```python
from build123d import *

# Parameters (mm, degrees)
PAD_DEPTH    = 5
SKETCH002_W  = 180
SKETCH002_H  = 5
PAD002_DEPTH = 5
PAD003_DEPTH = 10


with BuildPart() as part:
    # Sketch → Pad (new body)
    with BuildSketch(Plane.XY):
        with BuildLine():
            Line((0, 0), (-11.5, 0))
            ThreePointArc((-13.5, 2), (-12.914214, 0.585786), (-11.5, 0))
            Line((-13.5, 2), (-13.5, 7))
            ThreePointArc((-12, 7), (-12.75, 7.75), (-13.5, 7))
            Line((-12, 7), (-12, 3))
            ThreePointArc((-12, 3), (-11.707107, 2.292893), (-11, 2))
            Line((-11, 2), (-3, 2))
            ThreePointArc((-3, 2), (-2.292893, 2.292893), (-2, 3))
            Line((-2, 8), (-2, 3))
            ThreePointArc((-2, 8), (-2.292893, 8.707107), (-3, 9))
            Line((-3, 9), (-9, 9))
            ThreePointArc((-9, 11), (-10, 10), (-9, 9))
            Line((0, 11), (-9, 11))
            Line((0, 11), (0, 0))
        make_face()
    extrude(amount=PAD_DEPTH)

    # Sketch002 → Pad002 (join)
    with BuildSketch(Plane.XY):
        with Locations((90, 2.5)):
            Rectangle(SKETCH002_W, SKETCH002_H)
    extrude(amount=PAD002_DEPTH)

    # Sketch001 → Pad003 (join)
    with BuildSketch(Plane(origin=(180, 0, 0), x_dir=(-1, 0, 0), z_dir=(0, 0, -1))):
        with BuildLine():
            Line((0, 0), (-39.499167, 0))
            Line((-39.499167, 0), (-39.499167, 2.1))
            Line((-39.499167, 2.1), (-39.499167, 7.6))
            Line((-39.499167, 7.6), (-37.101251, 7.6))
            ThreePointArc((-33.5, 2), (-34.452609, 5.345343), (-37.101251, 7.6))
            Line((-33.5, 2), (-2, 2))
            Line((-2, 2), (-2, 15))
            Line((-2, 15), (-10, 15))
            Line((-10, 15), (-10, 17))
            Line((-10, 17), (0, 17))
            Line((0, 17), (0, 0))
        make_face()
    extrude(amount=-PAD003_DEPTH)


solid = part.part
```
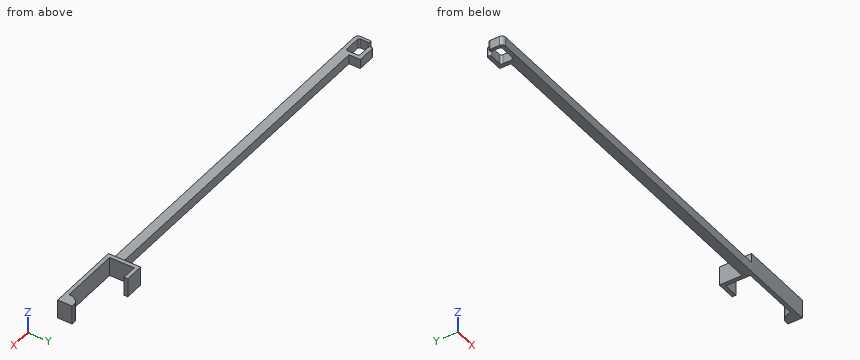
CAD build for the part. Positions are in the model's coordinates, mm. Coordinates: 2 decimals unless noted, no trailing zeros. Write each loop counter-clockwise with the first axis right and the second up, starting at its lowest first coordinate (ties: lowest second). Pieces come first, ordered by that corner, then holes. Notation, with made-up numbers: (38.5, -5) -> (92.5, -5) arc R14 ccw to (92.5, 11) -> close; hole circle Ø11 at (-8.75, 6.25). An arc over 180 degrees is marked (long way). Return JSON: item names as keys, results as strings. Group by question number.
Q1. Flat gauge pins, fed straight in: pin 1 (5 mm diameter, centred on x = 92.5, z = 6.5, fed in from +Y); pin 2 (1.5 mm diameter, centred on y = 12.5, z = 7.5, fed in from -X); pin 3 (5.5 mm diameter, centred on x = -8, z = 2.5, fed in from +Y). Where does each tip first touch, or does it go through?
Q2. Cut at A-A, the plane z = 7.5. Give the cut face in (x, y), then the cut area to 3 significant figures.
Q3. Cut at B-B, the plane x = 45. Give the cut face in (y, z), then the cut area to 3 significant figures.
Q4. Drill centre lines: line 1 (X direction, y = 2.75, z = 4.25); line 2 (X direction, y = 2.25, z = 1.25); line 3 (Y direction, x = 85.5, z = 2.5). Where is each one in solid material? Low to high.
Returned:
{
 "1": {"pin 1": "stops at y = 5", "pin 2": "stops at x = 180", "pin 3": "stops at y = 11"},
 "2": {"outline": "(180, 0) -> (219.5, 0) -> (219.5, 7.6) -> (217.1, 7.6) arc R6 ccw to (213.5, 2) -> (182, 2) -> (182, 15) -> (190, 15) -> (190, 17) -> (180, 17) -> close", "area": "153 mm2"},
 "3": {"outline": "(0, 0) -> (5, 0) -> (5, 5) -> (0, 5) -> close", "area": "25.0 mm2"},
 "4": {"line 1": "x = -13.5 to -11.97, -2.03 to 182, 213.53 to 219.5", "line 2": "x = -13.5 to -11.66, -2.34 to 182, 213.5 to 219.5", "line 3": "y = 0 to 5"}
}
